Autodesk Inventor part; units mm, degrees
ref_plane "YZ Plane" through (0, 0, 0) normal (1, 0, 0) x (0, 1, 0)
ref_plane "XZ Plane" through (0, 0, 0) normal (0, 1, 0) x (-1, 0, 0)
ref_plane "XY Plane" through (0, 0, 0) normal (0, 0, 1) x (1, 0, 0)
sketch "Esboço1" plane through (0, 0, 0) normal (0, 0, 1) x (1, 0, 0)
  circle A0 centre (-25.0665, 24.8448) radius 1.621
  circle A1 centre (24.9335, -25.1552) radius 1.621
  line L0 (-25.0665, 24.8448) -> (24.9335, -25.1552)
  line L1 (-33.0665, -33.1552) -> (32.9335, -33.1552)
  line L2 (32.9335, -33.1552) -> (32.9335, 32.8448)
  line L3 (32.9335, 32.8448) -> (-33.0665, 32.8448)
  line L4 (-33.0665, 32.8448) -> (-33.0665, -33.1552)
  line L5 (-33.0665, -33.1552) -> (32.9335, 32.8448) construction
  line L6 (32.9335, -33.1552) -> (-33.0665, 32.8448) construction
  circle A2 centre (-0.0665, -0.1552) radius 2.5192
  circle A3 centre (24.9335, 24.8448) radius 1.621
  circle A4 centre (-25.0665, -25.1552) radius 1.621
  point P0 (0, 0)
  dimension "d0" = 66
  dimension "d1" = 66
extrude "Extrusão1" add sketch "Esboço1" along normal blind 9.5
sketch "Esboço2" plane through (0, 0, 9.5) normal (0, 0, 1) x (1, 0, 0)
  circle A0 centre (24.9335, 24.8448) radius 1.621
  circle A1 centre (-25.0665, 24.8448) radius 1.621
  circle A2 centre (-25.0665, -25.1552) radius 1.621
  circle A3 centre (24.9335, -25.1552) radius 1.621
  point P0 (0, 0)
hole "Furo1" at (24.9335, 24.8448, 9.5) at (-25.0665, 24.8448, 9.5) at (-25.0665, -25.1552, 9.5) at (24.9335, -25.1552, 9.5) direction (0, 0, -1) diameter 4.5 end through all
sketch "Esboço3" plane through (0, 0, 9.5) normal (0, 0, 1) x (1, 0, 0)
  circle A0 centre (-0.0665, -0.1552) radius 2.5192
  point P0 (0, 0)
hole "Furo2" at (-0.0665, -0.1552, 9.5) direction (0, 0, -1) diameter 8.376 end through all
properties part number "Acoplador do pé nivelador"
Geometry check sheet. Reference: the model listing, model coordinates, mm. Round coordinates to 2 decimals unless told otherwise and drop trailing zeros. Write each loop counter-clockwise with the first axis right and the second up, starting at its lowest first coordinate (ties: lowest second). Pieces come first, ordered by that corner, then holes. Notation, with made-up numbers: (70, 4.5) -> (129, 4.5) arc R29 ccw to (129, 41.5) -> close; hole circle Ø3 at (15.5, -1). An arc over 180 degrees is marked (long way). One line per item, written item: value. Start each with the question number.
(1) Go/stop test with flat-tipped pins: pin 1 Ø4 at (x, y) = (-24, 9) entering from -Z; pin 2 Ø2.5 at (x, y) = (24.93, -25.16) entering from +Z. Record where each tip stops, or that it passes through.
(2) Cross-section at A-A, the plane z = 6. Record the cut outline in (x, y).
(3) Cross-section at C-C, the plane x = -1. Record the cut outline in (y, z), and give its area (3 significant figures).
(4) Scan lines: line 1 (Y direction, x = 0, z = 8.5); line 2 (X direction, y = 23, z = 5.5); line 3 (Y direction, x = 24, z = 4.25). Record each from-to range of solid material in increasing order. Write a range as [from, to].
(5) Draft check along X on faces 1 (the flat face through (32.934, -1, 5)), 2 (the cylindrical face through (-26.59, -23.5, 4.68)), 3 (the flat face through (0, 32.845, 5)). Enter one of: +X half, -X half, draft (parallel to the pull), parting line (faces both ways), or undercut.
(6) Cross-section at B-B, the plane y = 1. Record the cut outline in (x, z), and give its area (3 significant figures).
Answer:
1. pin 1: z = 0
1. pin 2: through
2. outline: (-33.07, -33.16) -> (32.93, -33.16) -> (32.93, 32.84) -> (-33.07, 32.84) -> close; hole circle Ø4.5 at (-25.07, -25.16); hole circle Ø4.5 at (-25.07, 24.84); hole circle Ø8.38 at (-0.07, -0.16); hole circle Ø4.5 at (24.93, -25.16); hole circle Ø4.5 at (24.93, 24.84)
3. outline: (-33.16, 0) -> (-4.24, 0) -> (-4.24, 9.5) -> (-33.16, 9.5) -> close; (3.93, 0) -> (32.84, 0) -> (32.84, 9.5) -> (3.93, 9.5) -> close
3. area: 549 mm²
4. line 1: [-33.16, -4.34], [4.03, 32.84]
4. line 2: [-33.07, -26.35], [-23.78, 23.65], [26.22, 32.93]
4. line 3: [-33.16, -27.2], [-23.11, 22.8], [26.89, 32.84]
5. face 1: +X half
5. face 2: undercut
5. face 3: draft
6. outline: (-33.07, 0) -> (-4.09, 0) -> (-4.09, 9.5) -> (-33.07, 9.5) -> close; (3.96, 0) -> (32.93, 0) -> (32.93, 9.5) -> (3.96, 9.5) -> close
6. area: 551 mm²
